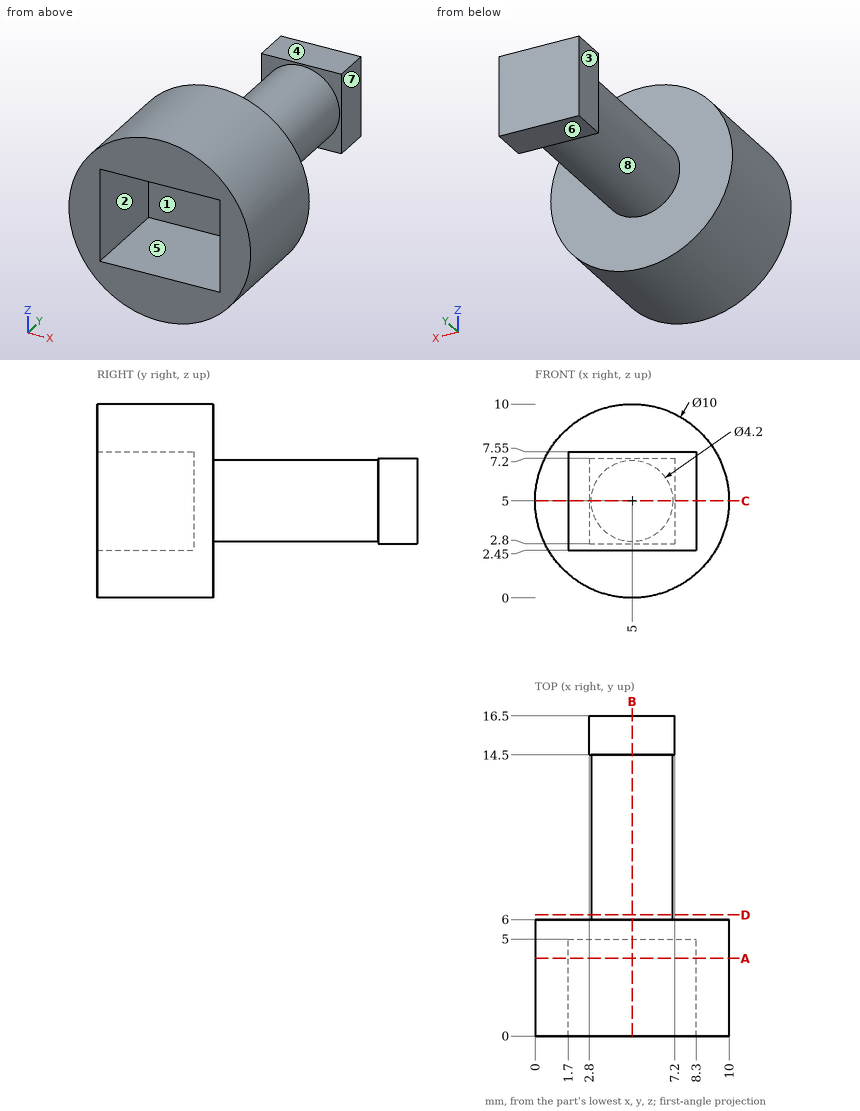
Design review of the part shown in the three views and the two pictorial views. Dimensions are in mm from the part's minimum x, y and z. A direction names the side the tool comes from. Round coordinates to 2 decimals unless told otherwise and drop trailing zeros. Loops run counter-clockwise (first coordinate to the right, second up) from the corner with the lowest first, then second, coordinate; pieces in that order, holes last.
Q1. Mouldability with a two-part tool opening along X and no side actions: class the marked faces 1, 2, 3 and 4 as +X half, -X half, draft (parallel to the pull), parting line (faces both ways), or undercut.
Result sheet:
face 1: undercut
face 2: undercut
face 3: -X half
face 4: draft
Q2. Add section B-B on x = 5. Write out the cut boundary in (y, z).
Result sheet:
outline: (0, 0) - (6, 0) - (6, 2.9) - (14.5, 2.9) - (14.5, 2.8) - (16.5, 2.8) - (16.5, 7.2) - (14.5, 7.2) - (14.5, 7.1) - (6, 7.1) - (6, 10) - (0, 10) - (0, 7.55) - (5, 7.55) - (5, 2.45) - (0, 2.45) - close
Q3. Insertion check: pin 1 Ø1.5 at (x, y) = (6, 3.5) entering from -Z; pin 2 Ø2 at (x, z) = (6, 3.5) entering from -Y; pin 3 Ø4 at (y, z) = (14.5, 5.5) entering from +X; pin 4 Ø4 at (x, z) = (6, 6) entering from -Y. Each pin has a flat end and moves straight along its axis. Give the tip position at first contact, or say it passes through.
Result sheet:
pin 1: stops at z = 0.01
pin 2: stops at y = 5
pin 3: stops at x = 7.2
pin 4: stops at y = 0
Q4. Add section C-C on z = 5. Write out the cut boundary in (x, y), plus the area to 3 significant figures.
Result sheet:
outline: (0, 0) - (1.7, 0) - (1.7, 5) - (8.3, 5) - (8.3, 0) - (10, 0) - (10, 6) - (7.1, 6) - (7.1, 14.5) - (7.2, 14.5) - (7.2, 16.5) - (2.8, 16.5) - (2.8, 14.5) - (2.9, 14.5) - (2.9, 6) - (0, 6) - close
area: 71.5 mm2
Q5. Add section A-A on y = 4. Write out the cut boundary in (x, z), plus the area to 3 significant figures.
Result sheet:
outline: circle Ø10 at (5, 5); hole (1.7, 2.45) - (8.3, 2.45) - (8.3, 7.55) - (1.7, 7.55) - close
area: 44.9 mm2
Q6. Add section D-D on y = 6.25. Write out the cut boundary in (x, z), plus the area to 3 significant figures.
Result sheet:
outline: circle Ø4.2 at (5, 5)
area: 13.9 mm2
Q7. Machinability: for the marked faces 5, 6, 7 and 8, which of the approach directions +Z, -Z, +X, -X, +Y, -Y give a long, thin tool a straight path to every point of the face, cutting with its end or side? Answer none if there is none.
Result sheet:
face 5: -Y
face 6: -Z, +X, -X, +Y
face 7: +Z, -Z, +X, +Y
face 8: none
Q8. To check wall thickness, follow line 1 along Y through (x, z) = (3.5, 3.25); line 2 along Z through (x, y) = (5, 14.25); line 3 along Y through (x, z) = (5, 2.5). State the ranges of each line that lie inside material, in increasing order.
Result sheet:
line 1: y = 5 to 6, 14.5 to 16.5
line 2: z = 2.9 to 7.1
line 3: y = 5 to 6
